Verification items for the finished model (mm, model axes). Round coordinates to 2 decimals unless told otherwise and drop trailing zeros. Order: outer loops, then holes, each group sorted by start corner. A loop starts at its lowest first (then second) coordinate and runs counter-clockwise, first axis right, second up. Notation, with made-up numbers: (27, 57) -> (50, 57) arc R26 cw to (50, 76) -> close; hole circle Ø5 at (-3, -0.5). An arc over 180 degrees is marked (long way). Put each result on its own line as item: value.
Autodesk Fusion 360 part; units mm, degrees
sketch "草图1" plane through (0, 0, 0) normal (0, 0, 1) x (1, 0, 0)
  circle A0 centre (0, 0) radius 21.5
  circle A1 centre (0, 0) radius 37.5 construction
  circle A2 centre (0, 0) radius 42.5
  line L0 (0, 0) -> (0, 56.853) construction
  circle A3 centre (0, 37.5) radius 1.65
  circle A4 centre (-24.1045, 28.7267) radius 1.65
  circle A5 centre (-36.9303, 6.5118) radius 1.65
  circle A6 centre (-32.476, -18.75) radius 1.65
  circle A7 centre (-12.8258, -35.2385) radius 1.65
  circle A8 centre (12.8258, -35.2385) radius 1.65
  circle A9 centre (32.476, -18.75) radius 1.65
  circle A10 centre (36.9303, 6.5118) radius 1.65
  circle A11 centre (24.1045, 28.7267) radius 1.65
  line L1 (0, 0) -> (0, -49) construction
  circle A12 centre (0, -29) radius 2.2361
  dimension "d1" = 43
  dimension "d2" = 75
  dimension "d3" = 85
  dimension "d4" = 3.3
  dimension "d6" = 360
  dimension "d8" = 29
extrude "拉伸1" add sketch "草图1" along normal blind 5
sketch "草图5" plane through (0, 0, 0) normal (0, 0, 1) x (1, 0, 0)
  circle A0 centre (-55, 20) radius 2.25
  circle A1 centre (-55, -20) radius 2.25
  circle A2 centre (-55, 20) radius 5.5
  circle A3 centre (-55, -20) radius 5.5
  circle A4 centre (0, 0) radius 42.5
  circle A5 centre (-61.2801, 100.2547) radius 75
  circle A6 centre (-61.2801, -100.2547) radius 75
  circle A7 centre (-101.3708, 0) radius 45
  dimension "d19" = 40
  dimension "d20" = 4.5
  dimension "d21" = 4.5
  dimension "d22" = 20
  dimension "d23" = 11
  dimension "d24" = 11
  dimension "d25" = 85
  dimension "d26" = 150
  dimension "d27" = 55
  dimension "d28" = 150
  dimension "d29" = 90
extrude "拉伸3" add sketch "草图5" along normal blind 5 contours A2 | A2 A3 A4 A5 A6 A7 | A3
Item 1: Gauge pin test, flat ends, axial feed: pin 1 Ø1.5 at (y, z) = (2, 2.5) entering from -X; pin 2 Ø6 at (x, y) = (0, -29) entering from -Z; pin 3 Ø2 at (y, z) = (-10, 3) entering from +X. Record the tip position at first contact, or that the pin passes through.
Check sheet entries:
pin 1: stops at x = -56.45
pin 2: stops at z = 0
pin 3: stops at x = 41.54
Item 2: Section check D-D on y = 37.5. Record the boundary of the cut face in (x, z), then the cut area to 4 significant figures.
Check sheet entries:
outline: (-20, 0) -> (-1.65, 0) -> (-1.65, 5) -> (-20, 5) -> close; (1.65, 0) -> (20, 0) -> (20, 5) -> (1.65, 5) -> close
area: 183.5 mm^2
Item 3: Section check B-B on x = 0. Record the boundary of the cut face in (y, z), then the cut area to 3 significant figures.
Check sheet entries:
outline: (-42.5, 0) -> (-31.24, 0) -> (-31.24, 5) -> (-42.5, 5) -> close; (-26.76, 0) -> (-21.5, 0) -> (-21.5, 5) -> (-26.76, 5) -> close; (21.5, 0) -> (35.85, 0) -> (35.85, 5) -> (21.5, 5) -> close; (39.15, 0) -> (42.5, 0) -> (42.5, 5) -> (39.15, 5) -> close
area: 171 mm^2
Item 4: Section check A-A on y = 0. Record the boundary of the cut face in (x, z).
Check sheet entries:
outline: (-56.37, 0) -> (-21.5, 0) -> (-21.5, 5) -> (-56.37, 5) -> close; (21.5, 0) -> (42.5, 0) -> (42.5, 5) -> (21.5, 5) -> close
Item 5: Material ranges on L1, parallel to Y at x = 0, z = 3.25; L2, parallel to Y at x = -53, z = 2.95; L3, parallel to Y at x = -55, z = 1.7, recorded low to high. Write a range as [from, to].
Check sheet entries:
L1: y = [-42.5, -31.24], [-26.76, -21.5], [21.5, 35.85], [39.15, 42.5]
L2: y = [-25.71, -21.03], [-18.97, 18.97], [21.03, 25.71]
L3: y = [-25.52, -22.25], [-17.75, 17.75], [22.25, 25.52]
Item 6: Section check C-C on z = 3.55. State how many separate pieces and enclosed holes the cut face has, then the cut area to 3 significant figures.
Check sheet entries:
separate pieces: 1
enclosed holes: 13
area: 5,150 mm^2
Item 7: Release check for a two-part mould opening along X. For faces 1 (the cylindrical face through (-56.37, 0.26, 2.46)), 2 (the cylindrical face through (42.48, 1.26, 2.46)), 3 (the cylindrical face through (35.28, 6.44, 2.46)) record: +X half, -X half, draft (parallel to the pull), parting line (faces both ways), or undercut.
Check sheet entries:
face 1: -X half
face 2: parting line
face 3: undercut
